Read the model definition and answer for the solid it produces. Units are mm, in the model's axes. Face numbers are marked on the shaded views. A direction names the side the tool comes from. Coordinates: 2 decimals unless noted, no trailing zeros. Write each loop counter-clockwise with the first axis right and the second up, starting at its lowest first coordinate (ties: lowest second). Pieces come first, ordered by that corner, then holes. Notation, with made-up numbers: (68.5, 47) -> (113.5, 47) arc R21 ccw to (113.5, 79) -> close; hole circle Ø6 at (27.5, -14.5). An arc over 180 degrees is marked (long way). Write item = value, one per line. Start each with the question number.
1) Section A-A (x = 10) is taken. Determine the outline of the cut face in (y, z).
2) For a pull along X with two mould halves and no side action, classify the marked faces 1, 2 and 3 as released by +X, released by -X, zero draft, split by the parting line, or undercut.
3) A tool of negligible diameter and unlimited length cuts with its end or side. For the marked faces 4, 5 and 6, from which of +Z, -Z, +X, -X, +Y, -Y can it reach the whole face along a straight path? Write none if from no direction.
4) Section B-B (z = 10) is taken. Determine the outline of the cut face in (x, y).
5) Flat-ended cylindrical pins translate along their axes: pin 1 Ø4 at (x, z) = (10, 10) entering from +Y; pin 2 Ø1 at (x, z) = (13.5, 6.5) entering from -Y; pin 3 Ø0.8 at (y, z) = (-0.5, 5.5) entering from -X; pin 4 Ø4 at (y, z) = (15, 17.5) entering from -X. Find the tip coordinate at first contact, or state that the pin passes through.
6) Section D-D (z = 16.75) is taken. Determine the outline of the cut face in (x, y), plus the area to 3 significant figures.
7) Find the intervals of material crossed by line 1 along X through (y, z) = (16, 7.75); line 2 along Z through (x, y) = (8.75, 16.25); line 3 along Y through (x, z) = (3.5, 13.75), in increasing order. Write a range as from..to.
8) Section C-C (y = 10) is taken. Determine the outline of the cut face in (x, z), plus the area to 3 significant figures.
from build123d import *

# Parameters (mm, degrees)
SKETCH_1_W          = 20
SKETCH_1_H          = 20
REVOLVE_1_ANGLE     = 90
SKETCH_2_W          = 16
SKETCH_2_H          = 18
CUT_EXTRUDE_1_DEPTH = 30
SKETCH_3_W          = 16
SKETCH_3_H          = 18
EXTRUDE_1_DEPTH     = 3
SKETCH_4_R          = 21
SKETCH_4_R_2        = 20
CUT_EXTRUDE_2_DEPTH = 35.641016151
SKETCH_5_R          = 1.5
CUT_EXTRUDE_3_DEPTH = 35.641016151
SKETCH_6_W          = 5
SKETCH_6_H          = 20
EXTRUDE_2_DEPTH     = 0.7
SKETCH_7_R          = 1.5
CUT_EXTRUDE_4_DEPTH = 100


with BuildPart() as part:
    # Эскиз1 → Повернуть1 (revolve)
    with BuildSketch(Plane.XY):
        with Locations((10, 10)):
            Rectangle(SKETCH_1_W, SKETCH_1_H)
    revolve(axis=Axis((0, 0, 0), (1, 0, 0)), revolution_arc=REVOLVE_1_ANGLE)

    # Эскиз2 → Вырез-Вытянуть1 (cut)
    with BuildSketch(Plane.XZ):
        with Locations((10, 11)):
            Rectangle(SKETCH_2_W, SKETCH_2_H)
    extrude(amount=-CUT_EXTRUDE_1_DEPTH, mode=Mode.SUBTRACT)

    # Эскиз3 → Бобышка-Вытянуть1 (add)
    with BuildSketch(Plane.XZ):
        with Locations((10, 11)):
            Rectangle(SKETCH_3_W, SKETCH_3_H)
    extrude(amount=-EXTRUDE_1_DEPTH)

    # Эскиз4 → Вырез-Вытянуть2 (cut, through all)
    with BuildSketch(Plane.ZY):
        Circle(SKETCH_4_R)
        Circle(SKETCH_4_R_2, mode=Mode.SUBTRACT)
    extrude(amount=-CUT_EXTRUDE_2_DEPTH, mode=Mode.SUBTRACT)

    # Эскиз5 → Вырез-Вытянуть3 (cut, through all)
    with BuildSketch(Plane(origin=(0, 0, 0), x_dir=(-1, 0, 0), z_dir=(0, 0, -1))):
        with Locations((-10, 10)):
            Circle(SKETCH_5_R)
    extrude(amount=-CUT_EXTRUDE_3_DEPTH, mode=Mode.SUBTRACT)

    # Эскиз6 → Бобышка-Вытянуть2 (add)
    with BuildSketch(Plane.XZ):
        with Locations((10, 10)):
            Rectangle(SKETCH_6_W, SKETCH_6_H)
    extrude(amount=EXTRUDE_2_DEPTH)

    # Эскиз7 → Вырез-Вытянуть4 (cut)
    with BuildSketch(Plane.XZ.offset(0.7)):
        with Locations(Location((10, 10, 0), (0, 0, 270))):
            Circle(SKETCH_7_R)
    extrude(amount=-CUT_EXTRUDE_4_DEPTH, mode=Mode.SUBTRACT)


solid = part.part
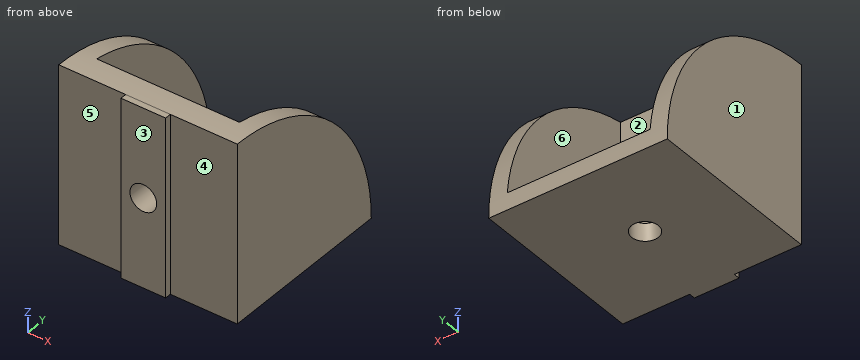
Answer key:
q1.outline = (-0.7, 0) -> (8.5, 0) -> (8.5, 2) -> (3, 2) -> (3, 8.5) -> (-0.7, 8.5) -> close; (-0.7, 11.5) -> (3, 11.5) -> (3, 19.77) arc R20 ccw to (0, 20) -> (-0.7, 20) -> close; (11.5, 0) -> (20, 0) arc R20 ccw to (19.9, 2) -> (11.5, 2) -> close
q2.face_1 = released by -X
q2.face_2 = undercut
q2.face_3 = zero draft
q3.face_4 = +Z, -Z, +X, -Y
q3.face_5 = +Z, -Z, -X, -Y
q3.face_6 = +Z, +Y
q4.outline = (0, 0) -> (7.5, 0) -> (7.5, -0.7) -> (8.5, -0.7) -> (8.5, 3) -> (2, 3) -> (2, 17.32) -> (0, 17.32) -> close; (11.5, -0.7) -> (12.5, -0.7) -> (12.5, 0) -> (20, 0) -> (20, 17.32) -> (18, 17.32) -> (18, 3) -> (11.5, 3) -> close
q5.pin_1 = 3
q5.pin_2 = 0
q5.pin_3 = 7.5
q5.pin_4 = through
q6.outline = (0, 0) -> (7.5, 0) -> (7.5, -0.7) -> (12.5, -0.7) -> (12.5, 0) -> (20, 0) -> (20, 10.93) -> (18, 10.93) -> (18, 3) -> (2, 3) -> (2, 10.93) -> (0, 10.93) -> close
q6.area = 95.2 mm^2
q7.line_1 = 0..2, 18..20
q7.line_2 = 0..2
q7.line_3 = 0..3
q8.outline = (0, 0) -> (8.5, 0) -> (8.5, 2) -> (2, 2) -> (2, 17.32) -> (0, 17.32) -> close; (11.5, 0) -> (20, 0) -> (20, 17.32) -> (18, 17.32) -> (18, 2) -> (11.5, 2) -> close
q8.area = 95.3 mm^2
